Geometry: final body of the model. Coordinates: model frame, mm. Round coordinates to 2 decimals unless told otherwise and drop trailing zeros. Order: outer loops, then holes, each group sorted by start corner. A loop starts at its lowest first (then second) coordinate and runs counter-clockwise, first axis right, second up. Notation, with made-up numbers: (85.5, 5.25) - (101.5, 5.25) arc R34 ccw to (101.5, 43.25) - close; hole circle Ø1 at (-39.75, 71.25). An arc over 180 degrees is marked (long way). Put each result on its own line as item: value. Start each with the question number.
(1) Material intervals for L1, parallel to Y at x = 3.5, z = 0.2; L2, parallel to Y at x = 7.5, z = 2.9; L3, parallel to X at y = 5, z = 0.6, sorted ascending. Write a range as [from, to].
(2) Section B-B (x = 3). Output: boundary loops of the cut face in (y, z).
(3) Section D-D (x = -13). Output: boundary loops of the cut face in (y, z), and give its area (3 significant figures).
(4) Pin query (flat end, axial travel): P1, Ø4, axis at x = -19.5, y = 33, coming from the +Z side; P2, Ø1, axis at y = 36, z = 0.5, coming from the -X side. Return the tip coordinate at first contact, or that it passes through.
(5) Pull-direction query (X, two-part tool) for faces 1 (the face through (5.13, 3.087, 1.503)), 2 (the face through (-4, 56, 2)), 3 (the face through (14.497, 28, 2)); classes: released by +X, released by -X, zero draft, split by the parting line, or undercut.
(6) Section C-C (z = 2). Output: boundary loops of the cut face in (x, y) (3 decimals), and give its area (3 significant figures).
(7) Section A-A (y = 28). Output: boundary loops of the cut face in (x, z), and give its area (3 significant figures).
Autodesk Inventor part; units mm, degrees
ref_plane "YZ Plane" through (0, 0, 0) normal (1, 0, 0) x (0, 1, 0)
ref_plane "XZ Plane" through (0, 0, 0) normal (0, 1, 0) x (-1, 0, 0)
ref_plane "XY Plane" through (0, 0, 0) normal (0, 0, 1) x (1, 0, 0)
sketch "Sketch1" plane through (0, 0, 0) normal (0, 0, 1) x (1, 0, 0)
  line L0 (-50.8, 101.6) -> (101.6, 101.6)
  line L1 (50.8, 0) -> (101.6, 101.6)
  line L2 (-28, 56) -> (0, 0)
  line L3 (14.6239, 7) -> (34.6239, 7)
  line L4 (34.6239, 7) -> (34.6239, 2)
  line L5 (34.6239, 2) -> (14.6239, 2)
  line L6 (14.6239, 2) -> (14.6239, 7)
  line L7 (50.8, 0) -> (50.8, 62.4863)
  line L8 (14.6239, 14) -> (34.6239, 14)
  line L9 (34.6239, 14) -> (34.6239, 9)
  line L10 (34.6239, 9) -> (14.6239, 9)
  line L11 (14.6239, 9) -> (14.6239, 14)
  line L12 (14.6239, 21) -> (34.6239, 21)
  line L13 (34.6239, 21) -> (34.6239, 16)
  line L14 (34.6239, 16) -> (14.6239, 16)
  line L15 (14.6239, 16) -> (14.6239, 21)
  line L16 (14.6239, 28) -> (34.6239, 28)
  line L17 (34.6239, 28) -> (34.6239, 23)
  line L18 (34.6239, 23) -> (14.6239, 23)
  line L19 (14.6239, 23) -> (14.6239, 28)
  line L20 (14.6239, 35) -> (34.6239, 35)
  line L21 (34.6239, 35) -> (34.6239, 30)
  line L22 (34.6239, 30) -> (14.6239, 30)
  line L23 (14.6239, 30) -> (14.6239, 35)
  line L24 (14.6239, 42) -> (34.6239, 42)
  line L25 (34.6239, 42) -> (34.6239, 37)
  line L26 (34.6239, 37) -> (14.6239, 37)
  line L27 (14.6239, 37) -> (14.6239, 42)
  circle A0 centre (43.7057, 6.2222) radius 3.1623
  circle A1 centre (43.7057, 28) radius 3.1623
  circle A2 centre (43.7057, 49.7778) radius 3.1623
  line L28 (24.6239, 0) -> (24.6239, -15.6085)
  circle A3 centre (5.5421, 49.7778) radius 3.1623
  circle A4 centre (5.5421, 6.2222) radius 3.1623
  circle A5 centre (5.5421, 28) radius 3.1623
  line L29 (34.6239, 44) -> (14.6239, 44)
  line L30 (14.6239, 44) -> (14.6239, 49)
  line L31 (34.6239, 49) -> (34.6239, 44)
  line L32 (14.6239, 49) -> (34.6239, 49)
  line L33 (34.6239, 51) -> (14.6239, 51)
  line L34 (14.6239, 51) -> (14.6239, 56)
  line L35 (14.6239, 56) -> (34.6239, 56)
  line L36 (34.6239, 56) -> (34.6239, 51)
  circle A6 centre (-34.29, 91.44) radius 3.1623
  circle A7 centre (85.09, 91.44) radius 3.1623
  line L37 (14.6239, 0) -> (-28, 0)
  line L38 (-28, 0) -> (-28, 56)
  line L39 (-28, 56) -> (14.6239, 56)
  line L40 (14.6239, 56) -> (14.6239, 0)
  line L41 (-28, 56) -> (0, 0)
  line L42 (-28, 56) -> (14.6239, 56)
  line L43 (14.6239, 56) -> (14.6239, 0)
  line L44 (14.6239, 0) -> (0, 0)
  line L45 (0, 0) -> (14.6239, 0)
  line L46 (34.6239, 0) -> (50.8, 0)
  dimension "d8" = 50.8
  dimension "d9" = 152.4
  dimension "d11" = 50.8
  dimension "d12" = 20
  dimension "d13" = 5
  dimension "d15" = 7
  dimension "d16" = 6.3246
  dimension "d17" = 6.3246
  dimension "d18" = 6.3246
  dimension "d19" = 14
  dimension "d21" = 6.2222
  dimension "d24" = 6.3246
  dimension "d25" = 6.3246
  dimension "d26" = 34.29
  dimension "d27" = 34.29
  dimension "d28" = 10.16
  dimension "d29" = 10.16
  dimension "d40" = 9.0818
  dimension "d41" = 9.0818
  dimension "d42" = 9.0818
  dimension "d43" = 9.0818
  dimension "d44" = 9.0818
  dimension "d45" = 9.0818
  dimension "d46" = 26.1761
extrude "Plate1" add sketch "Sketch1" along normal blind 3.048 contours L39 L34 L40 L30 L27 L23 L19 L15 L11 L6 L37 L2
sketch "Sketch2" plane through (0, 0, 3.048) normal (0, 0, 1) x (1, 0, 0)
  line L0 (14.6239, 56) -> (14.6239, 0)
  line L1 (-28, 56) -> (14.6239, 56)
  line L2 (14.6239, 0) -> (14.4969, 0)
  line L3 (14.4969, 0) -> (14.4969, 56)
  line L4 (14.4969, 56) -> (14.6239, 56)
  line L5 (14.6239, 56) -> (14.6239, 0)
  dimension "d33" = 0.127
extrude "Cut1" cut sketch "Sketch2" against normal blind 3.048
fillet "Corner Round1" radius 6.35 1 edges at (0, 0, 1.524)
fillet "Corner Round1" radius 3.175 1 edges at (-28, 56, 1.524)
equation "\"d17\" = d16"
equation "\"d18\" = d17"
equation "\"d21\" = 0.111111 * d20"
equation "\"d27\" = d26"
equation "\"d29\" = d28"
equation "\"d41\" = d40"
equation "\"d42\" = d40"
equation "\"d43\" = d42"
equation "\"d34\" = Thickness"
equation "\"BendRadius\" = Thickness"
equation "\"BendReliefWidth\" = Thickness"
equation "\"BendReliefDepth\" = 0.5 * Thickness"
equation "\"CornerReliefSize\" = 4 * Thickness"
equation "\"MinimumRemnant\" = 2 * Thickness"
equation "\"TransitionRadius\" = BendRadius"
equation "\"JacobiRadiusSize\" = BendRadius"
equation "\"GapSize\" = Thickness"
equation "\"d22\" = d21"
equation "\"d23\" = 0.5 * d20"
equation "\"d32\" = BendRadius"
properties part number "Belt plate mid"
Checks:
1. L1: y = [0.01, 3.81], [8.64, 25.59], [30.41, 47.36], [52.19, 56]
1. L2: y = [0, 3.74], [8.71, 25.52], [30.48, 47.29], [52.26, 56]
1. L3: x = [-2.5, 2.63], [8.46, 14.5]
2. outline: (0.07, 0) - (4.34, 0) - (4.34, 3.05) - (0.07, 3.05) - close; (8.1, 0) - (26.12, 0) - (26.12, 3.05) - (8.1, 3.05) - close; (29.88, 0) - (47.9, 0) - (47.9, 3.05) - (29.88, 3.05) - close; (51.66, 0) - (56, 0) - (56, 3.05) - (51.66, 3.05) - close
3. outline: (26, 0) - (56, 0) - (56, 3.05) - (26, 3.05) - close
3. area: 91.4 mm²
4. P1: passes through
4. P2: stops at x = -18.25
5. face 1: undercut
5. face 2: zero draft
5. face 3: released by +X
6. outline: (-25.703, 51.405) - (-1.755, 3.51) arc R6.35 ccw to (3.925, 0) - (14.497, 0) - (14.497, 56) - (-22.863, 56) arc R3.175 ccw to start; hole circle Ø6.325 at (5.542, 6.222); hole circle Ø6.325 at (5.542, 28); hole circle Ø6.325 at (5.542, 49.778)
6. area: 1,490 mm²
7. outline: (-14, 0) - (2.38, 0) - (2.38, 3.05) - (-14, 3.05) - close; (8.7, 0) - (14.5, 0) - (14.5, 3.05) - (8.7, 3.05) - close
7. area: 67.6 mm²
